Geometry: final body of the model. Coordinates: model frame, mm. Give positions to 0.01 mm unless a question says otherwise; leave off trailing zeros. Write each loop counter-clockwise with the first axis right and the second up, starting at its lowest first coordinate (ties: lowest second). Pieces come first, ordered by that corner, then holes. Notation, with made-up numbers: (-24.75, 57) -> (-14.75, 57) arc R29 cw to (-14.75, 94) -> close; hole circle Ø1 at (87.25, -24). An arc over 180 degrees is marked (long way). Use CSV: the item, a comma, the result in double quotes. Start each with the question number.
1) Material intervals for line 1 (Y direction, x = -10.5, z = 47.5); line 2 (Z direction, x = -30, y = -2); line 3 (Z direction, x = 40, y = -17.75), sorted ascending. Write a range as [from, to].
2) Section B-B (y = -11.25). Output: boundary loops of the cut face in (x, z), plus the area to 3 significant figures.
3) Section A-A (y = -18.25). Output: boundary loops of the cut face in (x, z), plus the area to 3 significant figures.
4) Contact query for flat-ended pins moving along their axis: P1, Ø6, axis at x = -17, y = -14.5, coming from the -Z side; P2, Ø10, axis at y = -13.5, z = -20, coming from the -X side; P3, Ø2, axis at y = -21, z = 0, coming from the -X side. Output: stop coordinate, or through.
```python
from build123d import *

# Parameters (mm, degrees)
F0_W     = 100.584
F0_H     = 123.444006
F1_DEPTH = 25.4
F2_R     = 20.849148
F3_R     = 5.08


with BuildPart() as f1:
    # F0 (on Front) → F1 (new body)
    with BuildSketch(Plane.XZ):
        with Locations((-2.4384, 0)):
            Rectangle(F0_W, F0_H)
    extrude(amount=F1_DEPTH)

    # F2
    f2_edges = [f1.edges().sort_by_distance(p)[0] for p in [
        (47.8536, -25.4, 0),
        (-2.4384, -25.4, 61.722003),
        (-52.7304, -25.4, 0),
        (-2.4384, -25.4, -61.722003),
    ]]
    fillet(f2_edges, radius=F2_R)

    # F3
    f3_edges = [f1.edges().sort_by_distance(p)[0] for p in [
        (47.8536, 0, 0),
        (-2.4384, 0, 61.722003),
        (-52.7304, 0, 0),
        (-2.4384, 0, -61.722003),
        (27.004452, -25.4, 0),
        (-2.4384, -25.4, -40.872855),
        (-2.4384, -25.4, 40.872855),
        (-31.881252, -25.4, 0),
    ]]
    fillet(f3_edges, radius=F3_R)


solid = f1.part
```
Answers follow:
1,line 1,"y = [-24.32, 0]"
1,line 2,"z = [-60.67, 60.67]"
1,line 3,"z = [-57.01, 57.01]"
2,outline,"(-51.62, -60.62) -> (46.75, -60.62) -> (46.75, 60.62) -> (-51.62, 60.62) -> close"
2,area,"11,900 mm^2"
3,outline,"(-47.6, -56.59) -> (42.72, -56.59) -> (42.72, 56.59) -> (-47.6, 56.59) -> close"
3,area,"10,200 mm^2"
4,P1,"stops at z = -60.53"
4,P2,"stops at x = -52.35"
4,P3,"stops at x = -45.88"
